Part print with two shaded views. Sizes in mm from the minimum x, y, z corner. Coordinates: 2 decimals unless noted, no trailing zeros. Order: outer loops, then holes, each group sorted by start corner. A loop starts at its lowest first (then second) coordinate and runs counter-clockwise, first axis right, second up. Notation, with made-up numbers: (13, 48) - (33, 48) arc R30 ccw to (33, 80) - close; hole circle Ø11 at (8.25, 87.25). An arc over 180 degrees is marked (long way). One line per item, written item: value.
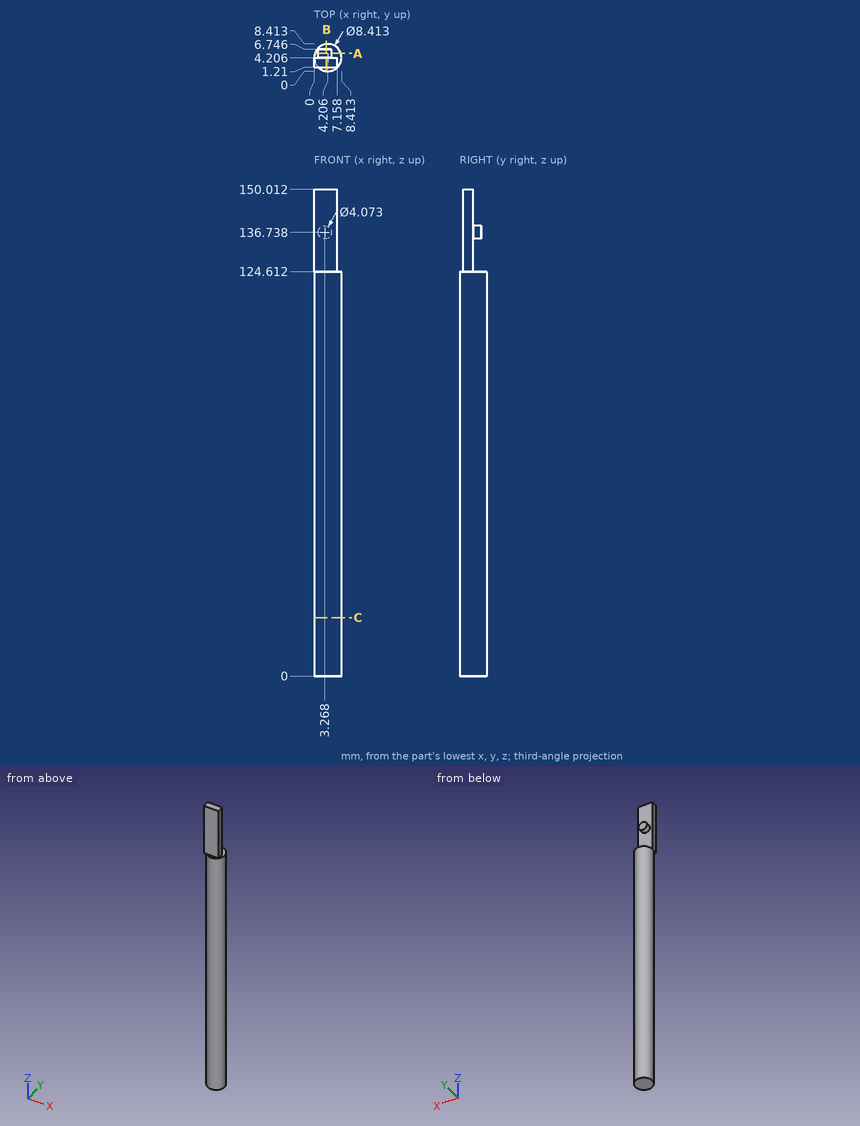
1. Band-saw the part on B-B, the plane x = 3.75. Give the cut face in (y, z) (1 decimal), and give its area (3 significant figures).
Values found:
outline: (0, 0) - (8.4, 0) - (8.4, 124.6) - (4.2, 124.6) - (4.2, 134.8) - (6.7, 134.8) - (6.7, 138.7) - (4.2, 138.7) - (4.2, 150) - (1.2, 150) - (1.2, 124.6) - (0, 124.6) - close
area: 1,130 mm2
2. Band-saw the part on C-C, the plane z = 18. Give the cut face in (x, y), and give its area (3 significant figures).
Values found:
outline: circle Ø8.41 at (4.21, 4.21)
area: 55.6 mm2
3. Flat gauge pins, fed straight in: P1, Ø0.6, axis at x = 0.5, y = 2.5, coming from the -Z side; P2, Ø3.5, axis at x = 3, z = 139.5, coming from the +Y side; P3, Ø1, axis at y = 7.5, z = 69.5, coming from the -X side; P4, Ø0.6, axis at x = 3, y = 0.5, coming from the +Z side. Where does each tip first touch, or does it go through?
Values found:
P1: stops at z = 0
P2: stops at y = 6.75
P3: stops at x = 1.06
P4: stops at z = 124.61
4. Probe line 1 along Z through (x, y) = (3, 6.5); line 2 along Z through (x, y) = (5, 1); line 3 along Y through (x, z) = (1, 137.5). List the from-to ranges inside material, lowest first.
Values found:
line 1: z = 0 to 124.61, 134.72 to 138.76
line 2: z = 0 to 124.61
line 3: y = 1.21 to 4.21
5. Band-saw the part on A-A, the plane y = 5.5. Give the cut face in (x, z).
Values found:
outline: (0.2, 0) - (8.21, 0) - (8.21, 124.61) - (0.2, 124.61) - close; circle Ø4.07 at (3.27, 136.74)
